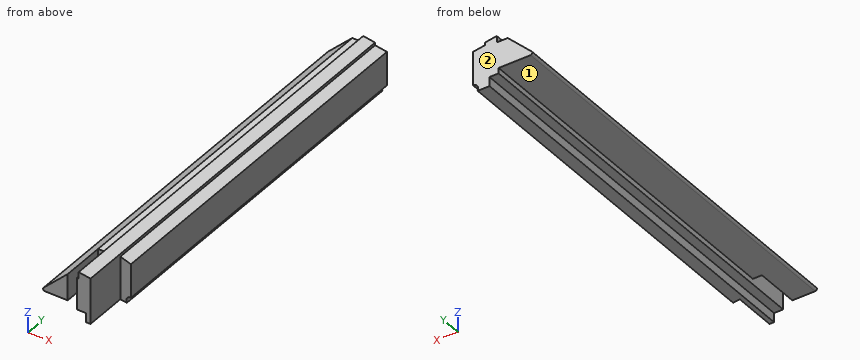
```python
from build123d import *

# Parameters (mm, degrees)
PAD005_DEPTH    = 450
POCKET002_DEPTH = 60
SKETCH011_W     = 10
SKETCH011_H     = 48
POCKET003_DEPTH = 60


with BuildPart() as part:
    # Sketch008 → Pad005 (new body)
    with BuildSketch(Plane.ZX):
        with BuildLine():
            Line((0, 0), (0, 12))
            Line((0, 12), (7, 12))
            Line((7, 12), (5, 25))
            Line((5, 25), (2, 25))
            Line((2, 25), (0, 38))
            Line((0, 38), (-37, 38))
            ThreePointArc((-45, 33), (-39.614381, 33.283009), (-37, 38))
            Line((-45, 33), (-45, 20))
            Line((-45, 20), (-35, 20))
            Line((-35, 20), (-35, 10))
            Line((-35, 10), (-29, 10))
            Line((-29, 10), (-29, -25.053428))
            ThreePointArc((-29, -25.053428), (-27.749682, -26.907606), (-25.562023, -26.443472))
            Line((-25.562023, -26.443472), (0, 0))
        make_face()
    extrude(amount=PAD005_DEPTH)

    # Sketch010 → Pocket002 (cut)
    with BuildSketch(Plane.XY.offset(10)):
        Polygon((25, 0), (25, 47.153846), (39, 45), (39, 0), align=None)
    extrude(amount=-POCKET002_DEPTH, mode=Mode.SUBTRACT)

    # Sketch011 → Pocket003 (cut)
    with BuildSketch(Plane.XY.offset(10)):
        with Locations((5, 24)):
            Rectangle(SKETCH011_W, SKETCH011_H)
    extrude(amount=-POCKET003_DEPTH, mode=Mode.SUBTRACT)


solid = part.part
```
Geometry check sheet. Reference: the model listing, model coordinates, mm. Face numbers are marked on the shaded views. Round coordinates to 2 decimals unless told otherwise and drop trailing zeros. Write each loop counter-clockwise with the first axis right and the second up, starting at its lowest first coordinate (ties: lowest second). Pieces come first, ordered by that corner, then holes. Notation, with made-up numbers: (12.25, 53) -> (52.25, 53) arc R25 cw to (52.25, 82) -> close; hole circle Ø8 at (69.5, 26). An arc over 180 degrees is marked (long way). Put each result on its own line as item: value.
1) Cross-section at B-B, the plane z = -8.5. Enter the section's corners in (x, y), plus the area to 3 significant figures.
Recorded:
outline: (-8.79, 0) -> (0, 0) -> (0, 48) -> (10, 48) -> (10, 0) -> (25, 0) -> (25, 47.15) -> (38, 45.15) -> (38, 450) -> (-8.79, 450) -> close
area: 20,000 mm2
2) Thickness scan on probe 1 along X at (y, z) = (376.5, -30); probe 2 along Z at (x, y) = (1, 342); probe 3 along X at (y, z) = (340, 4.5). Record the ranges inside material, lowest first. Write a range as from..to.
Recorded:
probe 1: x = 10..38
probe 2: z = -29..0
probe 3: x = 12..25
3) Cross-section at A-A, the plane y = 232.5. Enter the section's corners in (x, z) (1 decimal).
Recorded:
outline: (-26.4, -25.6) arc R2 ccw to (-25.1, -29) -> (10, -29) -> (10, -35) -> (20, -35) -> (20, -45) -> (33, -45) arc R5.6 cw to (38, -37) -> (38, 0) -> (25, 2) -> (25, 5) -> (12, 7) -> (12, 0) -> (0, 0) -> close
4) Cross-section at C-C, the plane x = -19. Enter the section's corners in (y, z).
Recorded:
outline: (0, -29) -> (450, -29) -> (450, -18.37) -> (0, -18.37) -> close
5) Depth check by flat-ended pin: P1, Ø8, axis at x = 12.5, y = 221, coming from the -Z side; P2, Ø6, axis at x = 8, y = 251.5, coming from the +Z side; P3, Ø8.5, axis at y = 13.5, z = -7.5, coming from the +X side. Enter the tip coordinate at first touch or a pass-through.
Recorded:
P1: stops at z = -35
P2: stops at z = 0
P3: stops at x = 25
6) Release check for a two-part mould opening along Y. For the marked faces 1 and 2 record: pulls with the +Y half, pulls with the -Y half, needs draft (parallel to the pull), parting line crosses it, or undercut.
Recorded:
face 1: needs draft
face 2: pulls with the +Y half
